from build123d import *

# Parameters (mm, degrees)
CROQUIS1_R              = 22.5
CROQUIS1_R_2            = 21
SALIENTE_EXTRUIR1_DEPTH = 785
CROQUIS2_W              = 10
CROQUIS2_H              = 60
CORTAR_EXTRUIR1_DEPTH   = 785


with BuildPart() as part:
    # Croquis1 → Saliente-Extruir1 (new body)
    with BuildSketch(Plane(origin=(0, 0, 0), x_dir=(1, 0, 0), z_dir=(0, 1, 0))):
        with Locations(Location((0, 0, 0), (0, 0, 270))):
            Circle(CROQUIS1_R)
        with Locations(Location((0, 0, 0), (0, 0, 270))):
            Circle(CROQUIS1_R_2, mode=Mode.SUBTRACT)
    extrude(amount=SALIENTE_EXTRUIR1_DEPTH)

    # Croquis2 → Cortar-Extruir1 (cut)
    with BuildSketch(Plane.XY):
        with Locations((0, 190)):
            Rectangle(CROQUIS2_W, CROQUIS2_H)
    extrude(amount=-CORTAR_EXTRUIR1_DEPTH, mode=Mode.SUBTRACT)


solid = part.part
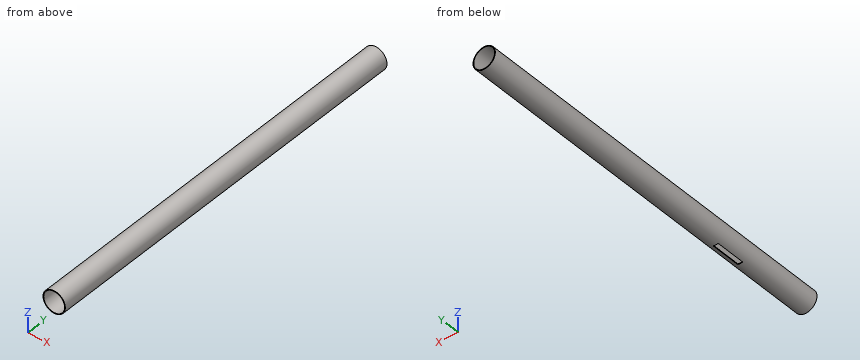
Work out the finished part from the listing and answer in its coordinate system (mm). Coordinates: 2 decimals unless noted, no trailing zeros. Write each loop counter-clockwise with the first axis right and the second up, starting at its lowest first coordinate (ties: lowest second). Pieces come first, ordered by that corner, then holes. Notation, with made-up numbers: M -19,-13.5 L -12,-13.5 A29 ccw -12,17.5 Z; hole C 82.5,50 d7. An arc over 180 degrees is marked long. Use one line per item in the form item = value. Start each with the question number.
1. The part is cut by section A-A (z = 0). Give the vertices of the cut face in (x, y).
2. The part is cut by section B-B (y = 437). Give the vertices of the cut face in (x, z), plus the area to 3 significant figures.
3. Each of these flat-tipped pins is pushed along its axis until it touches: P1, Ø10, axis at x = 9.5, z = 10.5, coming from the +Y side; P2, Ø5, axis at y = 696.5, z = 15.5, coming from the +X side; P3, Ø1, axis at y = 516, z = -13.5, coming from the -X side; P4, Ø1, axis at y = 658, z = 1.5, coming from the -X side. Where does it stop, or does it pass through?
4. Straight lines are drawn through the part: probe 1 along Z at (x, y) = (1, 80); probe 2 along X at (y, z) = (173.5, 0); probe 3 along X at (y, z) = (559, -1.5). For each, find the intervals that lie inside material, in ascending order. Write a range as from..to.
Evaluation:
q1.outline = M -22.5,0 L -21,0 L -21,785 L -22.5,785 Z; M 21,0 L 22.5,0 L 22.5,785 L 21,785 Z
q2.outline = C 0,0 d45; hole C 0,0 d42
q2.area = 205 mm^2
q3.P1 = through
q3.P2 = 18.36
q3.P3 = -18.36
q3.P4 = -22.48
q4.probe_1 = -22.48..-20.98, 20.98..22.48
q4.probe_2 = -22.5..-21, 21..22.5
q4.probe_3 = -22.45..-20.95, 20.95..22.45
